Part print with two shaded views. Sizes in mm from the minimum x, y, z corner. A direction names the side the tool comes from. Round coordinates to 2 decimals unless told otherwise and drop trailing zeros. Loops run counter-clockwise (first coordinate to the right, second up) from the corner with the lowest first, then second, coordinate; pieces in that order, holes last.
(1) Probe probe 1 along X at (y, z) = (5, 16.5) (1 decimal); probe 2 along Y at (x, z) = (4.25, 10); probe 3 along Y at (x, z) = (4.5, 20). List the from-to ranges inside material, lowest first.
(2) Flat gauge pins, fed straight in: pin 1 (1 mm diameter, centred on y = 8, z = 7.5, fed in from +X); pin 2 (1 mm diameter, centred on y = 6.5, z = 28.5, fed in from +X); pin 3 (3 mm diameter, centred on x = 4.76, y = 4.76, fed in from -Z). Where does each tip first touch, or does it go through?
(3) Cut at D-D on z = 22. List the corners of the cut face in (x, y) (1 decimal).
(4) Cut at A-A on z = 30.5. List the corners of the cut face in (x, y) (1 decimal).
(5) Cut at B-B on x = 1.5. List the corners of the cut face in (y, z) (1 decimal), then the cut area to 3 significant figures.
(6) Tool access for the marked faces 1 and 2: list every direction of +Z, -Z, +X, -X, +Y, -Y with a clear straight run to the whole face (end or side of a thin tool).
(7) Mould opens along X. For the marked faces 3, 4 and 5 say: +X half, -X half, draft (parallel to the pull), parting line (faces both ways), or undercut.
(8) Cut at C-C on y = 1.25. List the corners of the cut face in (x, z) (1 decimal).
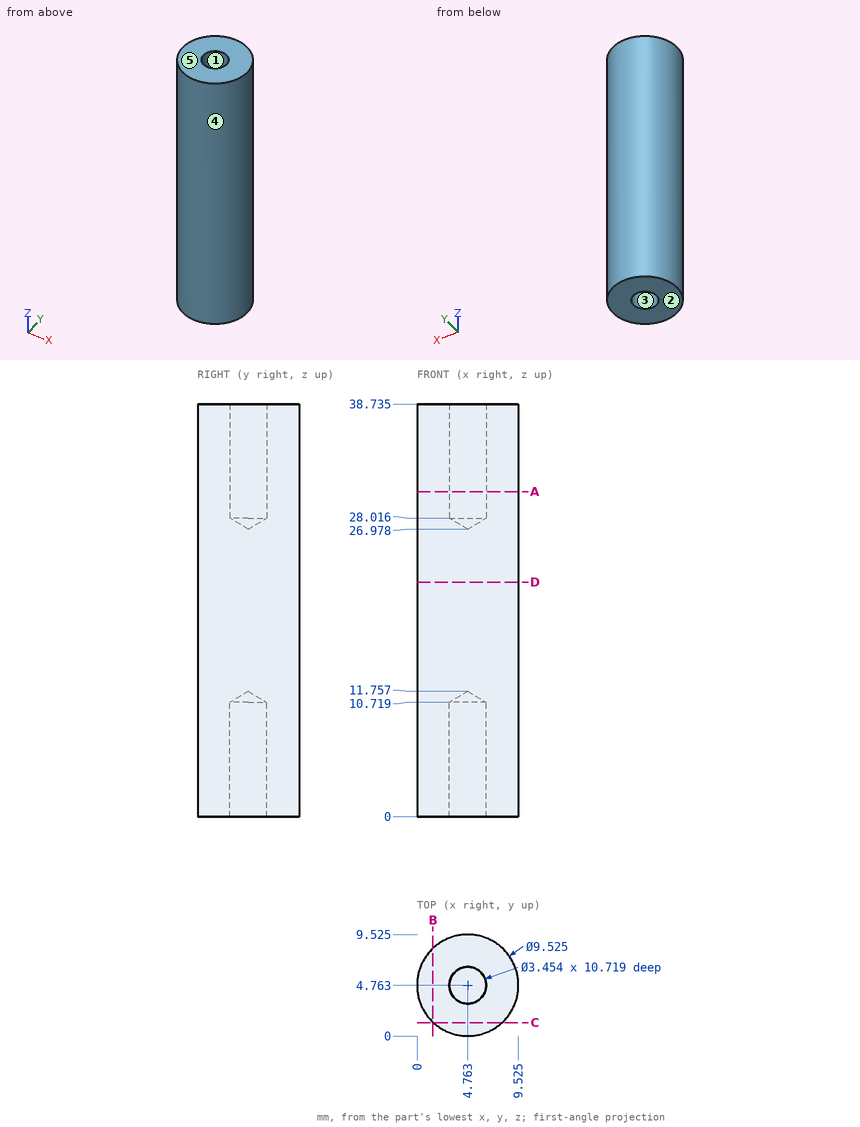
Final values:
1. probe 1: x = 0 to 9.5
1. probe 2: y = 0.03 to 3.11, 6.41 to 9.5
1. probe 3: y = 0.01 to 9.52
2. pin 1: stops at x = 8.66
2. pin 2: stops at x = 9.36
2. pin 3: stops at z = 10.85
3. outline: circle Ø9.5 at (4.8, 4.8)
4. outline: circle Ø9.5 at (4.8, 4.8); hole circle Ø3.5 at (4.8, 4.8)
5. outline: (1.3, 0) - (8.2, 0) - (8.2, 38.7) - (1.3, 38.7) - close
5. area: 269 mm2
6. face 1: +Z
6. face 2: -Z, +X, -X, +Y, -Y
7. face 3: undercut
7. face 4: parting line
7. face 5: draft
8. outline: (1.5, 0) - (8, 0) - (8, 38.7) - (1.5, 38.7) - close
